CAD build for the part. Positions are in the model's coordinates, mm. Face numbers are marked on the shaded views. A direction names the side the tool comes from. Coordinates: 2 decimals unless noted, no trailing zeros. Write each loop counter-clockwise with the first axis right and the second up, starting at its lowest first coordinate (ties: lowest second). Pieces come first, ordered by that corner, then holes. Notation, with made-up numbers: M 82.25,40 L 98.25,40 A20 ccw 98.25,61 Z; hole C -6,48 d3. An arc over 180 degrees is marked long. Put each result on its own line as item: value. Start each with the question number.
```python
from build123d import *

# Parameters (mm, degrees)
BOSS_EXTRUDE1_OUTLINE_W   = 120
BOSS_EXTRUDE1_OUTLINE_H   = 72
BOSS_EXTRUDE1_OUTLINE_W_2 = 104
BOSS_EXTRUDE1_OUTLINE_H_2 = 56
BOSS_EXTRUDE1_DEPTH       = 8
SKETCH3_W                 = 16
SKETCH3_H                 = 8
BOSS_EXTRUDE2_DEPTH       = 8
SKETCH4_W                 = 8
SKETCH4_H                 = 8
BOSS_EXTRUDE3_DEPTH       = 110
SKETCH5_W                 = 16
SKETCH5_H                 = 8
BOSS_EXTRUDE4_DEPTH       = 8
SKETCH6_R                 = 1.55
CUT_EXTRUDE1_DEPTH        = 211


# Read off the part's stored shape, not the designer's step: Boss-Extrude1
with BuildPart() as part:
    # Boss-Extrude1 outline → Boss-Extrude1 (new body)
    with BuildSketch(Plane(origin=(0, 0, 0), x_dir=(1, 0, 0), z_dir=(0, 1, 0))):
        with Locations((49.44492245, 21.253637361)):
            Rectangle(BOSS_EXTRUDE1_OUTLINE_W, BOSS_EXTRUDE1_OUTLINE_H)
        with Locations((49.44492245, 21.253637361)):
            Rectangle(BOSS_EXTRUDE1_OUTLINE_W_2, BOSS_EXTRUDE1_OUTLINE_H_2, mode=Mode.SUBTRACT)
    extrude(amount=BOSS_EXTRUDE1_DEPTH)

    # Sketch3 → Boss-Extrude2 (add)
    with BuildSketch(Plane.ZY.offset(10.55507755)):
        Polygon((-97.253637361, 14), (-97.253637361, 22), (-57.253637361, 8), (-57.253637361, 0), align=None)
        with Locations((-105.253637361, 18)):
            Rectangle(SKETCH3_W, SKETCH3_H)
    extrude(amount=-BOSS_EXTRUDE2_DEPTH)

    # Sketch4 → Boss-Extrude3 (add)
    with BuildSketch(Plane(origin=(-2.55507755, 0, 0), x_dir=(0, 0, -1), z_dir=(1, 0, 0))):
        with Locations((109.253637361, 18)):
            Rectangle(SKETCH4_W, SKETCH4_H)
    extrude(amount=BOSS_EXTRUDE3_DEPTH)

    # Sketch5 → Boss-Extrude4 (add)
    with BuildSketch(Plane(origin=(109.44492245, 0, 0), x_dir=(0, 0, -1), z_dir=(1, 0, 0))):
        Polygon((57.253637361, 0), (97.253637361, 14), (97.253637361, 22), (57.253637361, 8), align=None)
        with Locations((105.253637361, 18)):
            Rectangle(SKETCH5_W, SKETCH5_H)
    extrude(amount=-BOSS_EXTRUDE4_DEPTH)

    # Sketch6 → Cut-Extrude1 (cut)
    with BuildSketch(Plane.ZY.offset(10.55507755)):
        with Locations((2.746362639, 4)):
            Circle(SKETCH6_R)
        with Locations((-45.253637361, 4)):
            Circle(SKETCH6_R)
        with Locations((-101.253637361, 18)):
            Circle(SKETCH6_R)
    extrude(amount=-CUT_EXTRUDE1_DEPTH, mode=Mode.SUBTRACT)


solid = part.part
```
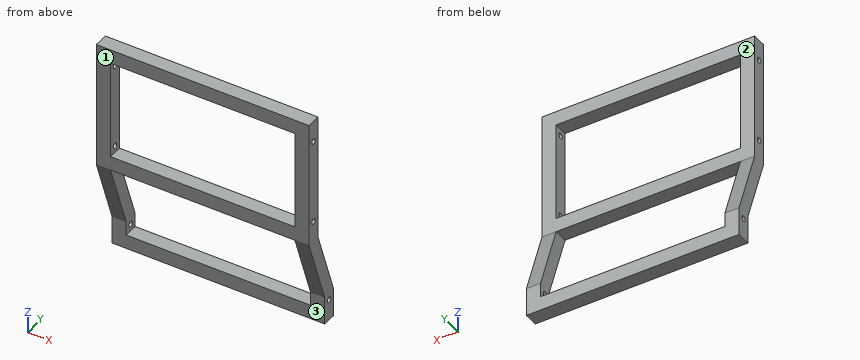
(1) Slice it at A-A, the plane z = -33. Write the cut outline in (x, y), then the cut area to 3 significant figures.
(2) Slice it at B-B, the plane x = 24. Write the cut outline in (y, z), then the cut area to 3 significant figures.
(3) Drill centre lines: line 1 (X direction, y = 5.25, z = -2.5); line 2 (Z direction, x = 7, y = 4); line 3 (Z direction, x = 77, y = 17). Where is each one in solid material? Low to high. Write a range as [from, to].
(4) Slice it at C-C, the plane y = 18. Write the cut outline in (x, z), then the cut area to 3 significant figures.
(5) Which spindle directions (+Z, -Z, +X, -X, +Y, -Y) get a long thin tool onto all of the face, cutting with end or side? Do the marked faces 1, 2 and 3. Say none if no direction does.
(6) Slice it at D-D, the plane y = 4. Write the cut outline in (x, z), then the cut area to 3 significant figures.
(7) Drop flat-ended pins along their axis: pin 1 (8 mm diameter, centred on x = 45, y = 12.5, fed in from +Z); pin 2 (5 mm diameter, centred on x = 61, z = -109, fed in from -Y); pin 3 (9 mm diameter, centred on x = 34.5, y = 2, fed in from -Z). Give the stop position or say it passes through.
Result set:
1. outline: M -10.56,0 L -2.56,0 L -2.56,8 L -10.56,8 Z; M 101.44,0 L 109.44,0 L 109.44,8 L 101.44,8 Z
1. area: 128 mm^2
2. outline: M 0,-57.25 L 8,-57.25 L 8,-49.25 L 0,-49.25 Z; M 0,6.75 L 8,6.75 L 8,14.75 L 0,14.75 Z; M 14,-113.25 L 22,-113.25 L 22,-105.25 L 14,-105.25 Z
2. area: 192 mm^2
3. line 1: x = [-10.56, -2.56], [101.44, 109.44]
3. line 2: z = [-57.25, -49.25], [6.75, 14.75]
3. line 3: z = [-113.25, -105.25]
4. outline: M -10.56,-113.25 L 109.44,-113.25 L 109.44,-102.8 L 101.44,-102.8 L 101.44,-105.25 L -2.56,-105.25 L -2.56,-102.8 L -10.56,-102.8 Z; M -10.56,-99.7 L -2.56,-99.7 L -2.56,-85.83 L -10.56,-85.83 Z; M 101.44,-99.7 L 109.44,-99.7 L 109.44,-85.83 L 101.44,-85.83 Z
4. area: 1,220 mm^2
5. face 1: +Z, -Z, +X, -X, -Y
5. face 2: +Z, +X, -X, +Y
5. face 3: -Z, +X, -X, -Y
6. outline: M -10.56,-68.68 L -2.56,-68.68 L -2.56,-57.25 L 101.44,-57.25 L 101.44,-68.68 L 109.44,-68.68 L 109.44,-46.8 L 101.44,-46.8 L 101.44,-49.25 L -2.56,-49.25 L -2.56,-46.8 L -10.56,-46.8 Z; M -10.56,-43.7 L -2.56,-43.7 L -2.56,1.2 L -10.56,1.2 Z; M -10.56,4.3 L -2.56,4.3 L -2.56,6.75 L 101.44,6.75 L 101.44,4.3 L 109.44,4.3 L 109.44,14.75 L -10.56,14.75 Z; M 101.44,-43.7 L 109.44,-43.7 L 109.44,1.2 L 101.44,1.2 Z
6. area: 2,900 mm^2
7. pin 1: stops at z = -105.25
7. pin 2: stops at y = 14
7. pin 3: stops at z = -57.25
